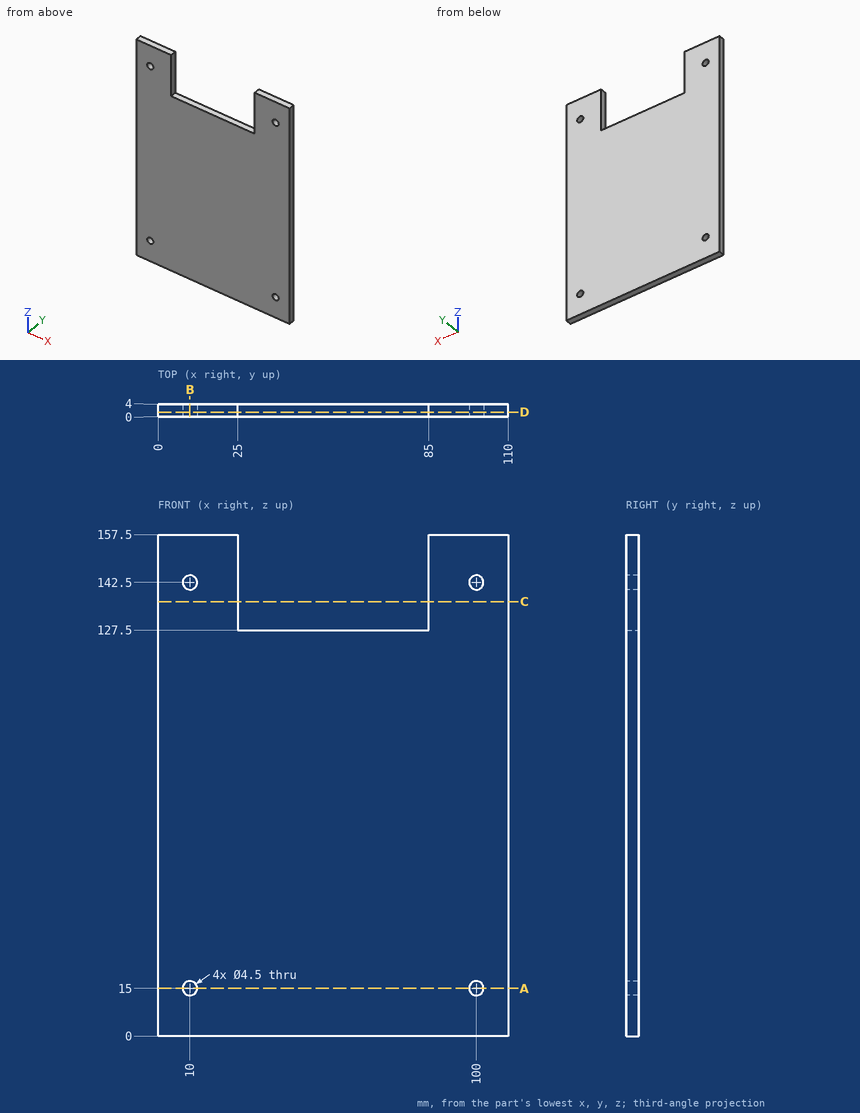
Geometry check sheet. Reference: drawing and pictorial views, mm from the part's lowest x, y, z. Give positions to 0.01 mm unless a question says otherwise; leave off trailing zeros. Loops run counter-clockwise (first coordinate to the right, second up) from the corner with the lowest first, then second, coordinate; pieces in that order, holes last. Notation, with made-up numbers: M 46.25,12.25 L 50.25,12.25 A28 cw 50.25,31.25 Z; hole C 75.5,51.5 d2. An arc over 180 degrees is marked long. Use a Markdown table: item, result. Add a question column.
Q1. Go/stop test with a flat-tipped pin: pin 1 (3.5 mm diameter, centred on x = 10, z = 142.5, fed in from -Y). Record where the tip stops, or that it passes through.
Q2. Sectioned sample at B-B, the plane x = 10. Record the cut outline in (y, z).
Q3. Sectioned sample at D-D, the plane y = 1.45. Record the cut outline in (x, z).
Q4. Scan lines: line 1 along X through (y, z) = (1.95, 142.5); line 2 along Z through (x, y) = (10, 1.1); line 3 along X through (y, z) = (1.75, 15). Record each from-to range of solid material in increasing order. Write a range as [from, to].
Q5. Sectioned sample at A-A, the plane z = 15. Record the cut outline in (x, y).
Q6. Sectioned sample at C-C, the plane z = 136.5. Record the cut outline in (x, y), then the cut area to 3 significant figures.
Verdict:
| question | item | result |
|---|---|---|
| 1 | pin 1 | through |
| 2 | outline | M 0,0 L 4,0 L 4,12.75 L 0,12.75 Z; M 0,17.25 L 4,17.25 L 4,140.25 L 0,140.25 Z; M 0,144.75 L 4,144.75 L 4,157.5 L 0,157.5 Z |
| 3 | outline | M 0,0 L 110,0 L 110,157.5 L 85,157.5 L 85,127.5 L 25,127.5 L 25,157.5 L 0,157.5 Z; hole C 10,15 d4.5; hole C 10,142.5 d4.5; hole C 100,15 d4.5; hole C 100,142.5 d4.5 |
| 4 | line 1 | [0, 7.75], [12.25, 25], [85, 97.75], [102.25, 110] |
| 4 | line 2 | [0, 12.75], [17.25, 140.25], [144.75, 157.5] |
| 4 | line 3 | [0, 7.75], [12.25, 97.75], [102.25, 110] |
| 5 | outline | M 0,0 L 7.75,0 L 7.75,4 L 0,4 Z; M 12.25,0 L 97.75,0 L 97.75,4 L 12.25,4 Z; M 102.25,0 L 110,0 L 110,4 L 102.25,4 Z |
| 6 | outline | M 0,0 L 25,0 L 25,4 L 0,4 Z; M 85,0 L 110,0 L 110,4 L 85,4 Z |
| 6 | area | 200 mm^2 |
